```python
from build123d import *

# Parameters (mm, degrees)
LOFT_2_DEPTH             = 20
LOFT_2_DRAFT             = -5.7105931
CUT_EXTRUDE_8_DEPTH      = 176.915490387
CUT_EXTRUDE_8_DEPTH_BACK = 176.915490387
FILLET_1_R               = 4
SHELL_1_T                = 2
CUT_EXTRUDE_9_DEPTH      = 2
SKETCH_15_R              = 3.1
EXTRUDE_2_DEPTH          = 3.1
SKETCH_16_W              = 12.261336097
SKETCH_16_H              = 9.48947362
SKETCH_16_R              = 3.1
EXTRUDE_3_DEPTH          = 3.1
HOLE_WIZARD_M2_1_D       = 1.6
HOLE_WIZARD_M2_1_DEPTH   = 2


# Read off the part's stored shape, not the designer's step: 放样2
with BuildPart() as part:
    # 放样2 outline → 放样2 (with draft: the straight prism first)
    with BuildSketch(Plane(origin=(0, -20, 0), x_dir=(1, 0, 0), z_dir=(0, 1, 0))):
        Polygon((2, -25.602070867), (82.579718414, -29.825074964), (169.852914921, -29.825074964), (169.852914921, 29.825074964), (82.579718414, 29.825074964), (2, 25.602070867), align=None)
    extrude(amount=LOFT_2_DEPTH)
    # 放样2: the draft: its side faces are tilted about the plane it starts from
    loft_2_sides = [part.faces().sort_by_distance(p)[0] for p in [
        (42.289859207, -10, 27.713572915),
        (126.216316668, -10, 29.825074964),
        (169.852914921, -10, 0),
        (126.216316667, -10, -29.825074964),
        (42.289859207, -10, -27.713572915),
        (2, -10, 0),
    ]]
    draft(loft_2_sides, Plane(origin=(0, -20, 0), x_dir=(1, 0, 0), z_dir=(0, 1, 0)), LOFT_2_DRAFT)

    # 草图8 → 切除-拉伸8 (cut, two sides: drawn at the far end of the back side and taken through both)
    with BuildSketch(Plane.XY.offset(-CUT_EXTRUDE_8_DEPTH_BACK)):
        Polygon((0, 0), (20, -20), (-19.267413558, -20), align=None)
    extrude(amount=CUT_EXTRUDE_8_DEPTH + CUT_EXTRUDE_8_DEPTH_BACK, mode=Mode.SUBTRACT)

    # 圆角1
    # the kernel refuses this fillet: 4 mm, written as the material it takes off along each edge
    with BuildSketch(Plane(origin=(82.580397323, -20.25926479, -29.799148485), x_dir=(-0.9986397137740413, 0.0025926566839660006, 0.0520768682297623), z_dir=(-0.002605587720042804, 0.9950338125721717, -0.09950338059946291))) as fillet_1_piece_1:
        with BuildLine():
            CenterArc((FILLET_1_R * 0.0260558773727, FILLET_1_R), FILLET_1_R, 267.014891807, 2.985108193)
            Line((-FILLET_1_R * 0.0260205222495, FILLET_1_R * 0.00135689628257), (0, 0))
            Line((0, 0), (FILLET_1_R * 0.0260558773727, 0))
        make_face()
    extrude(amount=20.620937018, mode=Mode.SUBTRACT)
    with BuildSketch(Plane(origin=(82.580397323, -20.25926479, 29.799148485), x_dir=(-0.9986397137740393, 0.002592656683969708, -0.05207686822979932), z_dir=(-0.002605587720042804, 0.9950338125721717, 0.09950338059946291))) as fillet_1_piece_2:
        with BuildLine():
            CenterArc((FILLET_1_R * 0.0260558773727, -FILLET_1_R), FILLET_1_R, 90, 2.985108193)
            Line((-FILLET_1_R * 0.0260205222495, -FILLET_1_R * 0.00135689628257), (0, 0))
            Line((0, 0), (FILLET_1_R * 0.0260558773727, 0))
        make_face()
    extrude(amount=20.620937018, mode=Mode.SUBTRACT)
    with BuildSketch(Plane(origin=(169.852914921, -20, 38.874950591), x_dir=(-1, 0, 0), z_dir=(0, 0, -1))) as fillet_1_piece_3:
        with BuildLine():
            CenterArc((FILLET_1_R * 0.904987562707, FILLET_1_R), FILLET_1_R, 185.7105931, 84.2894069)
            Line((-FILLET_1_R * 0.0900496275678, FILLET_1_R * 0.90049628163), (0, 0))
            Line((0, 0), (FILLET_1_R * 0.904987562707, 0))
        make_face()
    extrude(amount=77.749901182, mode=Mode.SUBTRACT)

    # 抽壳1 (no face opened: a closed hollow body)
    add(offset(amount=-SHELL_1_T, mode=Mode.PRIVATE), mode=Mode.SUBTRACT)

    # 草图11 → 切除-拉伸9 (cut)
    with BuildSketch(Plane(origin=(0, -20, 0), x_dir=(1, 0, 0), z_dir=(0, 1, 0))):
        with BuildLine():
            Line((32.7540299, 23.458252391), (26.119793836, 7.804096994))
            ThreePointArc((26.119793836, 7.804096994), (24.534355196, 0), (26.119793836, -7.804096994))
            Line((26.119793836, -7.804096994), (32.7540299, -23.458252391))
            Line((32.7540299, -23.458252391), (82.6670403, -27.825074964))
            Line((82.6670403, -27.825074964), (159.58071917, -27.825074964))
            Line((159.58071917, -27.825074964), (159.58071917, 27.825074964))
            Line((159.58071917, 27.825074964), (82.6670403, 27.825074964))
            Line((82.6670403, 27.825074964), (32.7540299, 23.458252391))
        make_face()
    extrude(amount=CUT_EXTRUDE_9_DEPTH, mode=Mode.SUBTRACT)

    # 草图15 → 凸台-拉伸2 (add)
    with BuildSketch(Plane.XZ.offset(2)):
        Polygon((72.850599149, 29.104930146), (60.999300983, 28.483829928), (60.999300983, 20.617464002), (72.850599149, 20.617464002), align=None)
        with Locations(Location((67.061317629, 25.566411224, 0), (0, 0, 73.416746399))):
            Circle(SKETCH_15_R, mode=Mode.SUBTRACT)
    extrude_2 = extrude(amount=EXTRUDE_2_DEPTH)

    # 镜向1: 凸台-拉伸2 across plane
    add(extrude_2.mirror(Plane(origin=(0, 0, 0), x_dir=(1, 0, 0), z_dir=(0, 0, -1))))

    # 草图16 → 凸台-拉伸3 (add)
    with BuildSketch(Plane.XZ.offset(2)):
        with Locations((150.788762168, 25.613857156)):
            Rectangle(SKETCH_16_W, SKETCH_16_H)
        with Locations(Location((150.788762168, 25.939901438, 0), (0, 0, 90))):
            Circle(SKETCH_16_R, mode=Mode.SUBTRACT)
    extrude_3 = extrude(amount=EXTRUDE_3_DEPTH)

    # 镜向2: 凸台-拉伸3 across plane
    add(extrude_3.mirror(Plane(origin=(0, 0, 0), x_dir=(1, 0, 0), z_dir=(0, 0, -1))))

    # M2 螺纹孔1
    with Locations(Plane(origin=(0, 0, 0), x_dir=(1, 0, 0), z_dir=(0, 1, 0))):
        with Locations((168.015540482, -27.047622993)):
            Hole(HOLE_WIZARD_M2_1_D / 2, depth=HOLE_WIZARD_M2_1_DEPTH)


solid = part.part
```
Verification items for the finished model (mm, model axes). A direction names the side the tool comes from. Round coordinates to 2 decimals unless told otherwise and drop trailing zeros. Loops run counter-clockwise (first coordinate to the right, second up) from the corner with the lowest first, then second, coordinate; pieces in that order, holes last. Notation, with made-up numbers: (-38, 74.5) -> (-1, 74.5) arc R18 ccw to (-1, 87.5) -> close; hole circle Ø5 at (21, 60.5). An arc over 180 degrees is marked (long way). Answer as a JSON object with one key per item and string values.
Q1. Access from +Z, -Z, +X, -X, +Y, -Y to the whole of each face (thin tool, end or side, straight path). Record for faces 1 (the flat face through (156.919, -4, 25)), 2 (the flat face through (58.06, -19.014, -25.672)), 3 (the flat face through (85, 0, 0)).
Data:
{"face 1": "none", "face 2": "-Y", "face 3": "+Z, -Z, +X, -X, +Y"}
Q2. Draft check along Z on faces 4 (the flat face through (72.851, -4, 25)), 5 (the cylindrical face through (168.947, -18.938, 0.423)), 6 (the flat face through (67, -2, 26)). Enter one of: pulls with the +Z half, pulls with the -Z half, needs draft (parallel to the pull), parting line crosses it, or undercut.
Data:
{"face 4": "undercut", "face 5": "needs draft", "face 6": "undercut"}
Q3. Go/stop test with flat-tipped pins: P1, Ø4, axis at y = -5.5, z = 2.5, coming from the -X side; P2, Ø1.6, axis at y = -4, z = -25, coming from the -X side; P3, Ø12, axis at x = 34, y = -6.5, coming from the +Z side. Record where each tip stops, or that it passes through.
Data:
{"P1": "stops at x = 3.5", "P2": "stops at x = 3.2", "P3": "stops at z = 29.31"}
Q4. Section check D-D (z = 12). Record the boundary of the cut face in (x, y).
Data:
{"outline": "(0, 0) -> (20, -20) -> (27.9, -20) -> (27.9, -18) -> (20.83, -18) -> (4.83, -2) -> (169.64, -2) -> (168.22, -16.2) arc R2 cw to (166.23, -18) -> (159.58, -18) -> (159.58, -20) -> (166.23, -20) arc R4 ccw to (170.21, -16.4) -> (171.85, 0) -> close"}
Q5. Section check A-A (x = 134). Record the boundary of the cut face in (y, z).
Data:
{"outline": "(-20, -29.83) -> (0, -31.83) -> (0, 31.83) -> (-20, 29.83) -> (-20, 27.83) -> (-18, 27.83) -> (-18, 28.02) -> (-2, 29.62) -> (-2, -29.62) -> (-18, -28.02) -> (-18, -27.83) -> (-20, -27.83) -> close"}
Q6. Section check B-B (z = 4). Record the boundary of the cut face in (x, y).
Data:
{"outline": "(0, 0) -> (20, -20) -> (24.94, -20) -> (24.94, -18) -> (20.83, -18) -> (4.83, -2) -> (169.64, -2) -> (168.22, -16.2) arc R2 cw to (166.23, -18) -> (159.58, -18) -> (159.58, -20) -> (166.23, -20) arc R4 ccw to (170.21, -16.4) -> (171.85, 0) -> close"}
Q7. Section check C-C (x = 37). Record the boundary of the cut face in (y, z).
Data:
{"outline": "(-20, -27.44) -> (0, -29.44) -> (0, 29.44) -> (-20, 27.44) -> (-20, 23.83) -> (-18, 23.83) -> (-18, 25.62) -> (-2, 27.23) -> (-2, -27.23) -> (-18, -25.62) -> (-18, -23.83) -> (-20, -23.83) -> close"}
Q8. Scan lines: line 1 (Y direction, x = 97, z = 12.5); line 2 (X direction, y = -17.75, z = 21); line 3 (Z direction, x = 68, y = -11.5). Record each from-to range of solid material in increasing order. Write a range as from..to.
Data:
{"line 1": "y = -2..0", "line 2": "x = 17.75..20.58, 167.2..169.83", "line 3": "z = -29.91..-27.9, 27.9..29.91"}
